```python
from build123d import *

# Parameters (mm, degrees)
SKETCH1_R           = 12.65
BOSS_EXTRUDE1_DEPTH = 4
SKETCH4_R           = 6
CUT_EXTRUDE3_DEPTH  = 0.5
SKETCH5_R           = 3
CUT_EXTRUDE4_DEPTH  = 1.5
FILLET1_R           = 0.5
FILLET2_R           = 0.5
FILLET3_R           = 0.5
SKETCH7_R           = 13.65
BOSS_EXTRUDE2_DEPTH = 1
SKETCH8_R           = 1.4
CUT_EXTRUDE6_DEPTH  = 20.941038087
CUT_EXTRUDE7_DEPTH  = 2.7
SKETCH16_R          = 1.65
CUT_EXTRUDE8_DEPTH  = 10


with BuildPart() as part:
    # Sketch1 → Boss-Extrude1 (new body)
    with BuildSketch(Plane(origin=(0, 0, 0), x_dir=(1, 0, 0), z_dir=(0, 1, 0))):
        with Locations(Location((0, 0, 0), (0, 0, 270))):
            Circle(SKETCH1_R)
    extrude(amount=BOSS_EXTRUDE1_DEPTH)

    # Sketch4 → Cut-Extrude3 (cut)
    with BuildSketch(Plane(origin=(0, 4, 0), x_dir=(1, 0, 0), z_dir=(0, 1, 0))):
        with Locations(Location((0, 0, 0), (0, 0, 270))):
            Circle(SKETCH4_R)
    extrude(amount=-CUT_EXTRUDE3_DEPTH, mode=Mode.SUBTRACT)

    # Sketch5 → Cut-Extrude4 (cut)
    with BuildSketch(Plane(origin=(0, 3.5, 0), x_dir=(1, 0, 0), z_dir=(0, 1, 0))):
        with Locations(Location((0, 0, 0), (0, 0, 270))):
            Circle(SKETCH5_R)
    extrude(amount=-CUT_EXTRUDE4_DEPTH, mode=Mode.SUBTRACT)

    # Fillet1
    fillet1_edges = [part.edges().sort_by_distance(p)[0] for p in [
        (0, 4, -6),
    ]]
    fillet(fillet1_edges, radius=FILLET1_R - 0.0001)  # a hair under: the kernel refuses the full size

    # Fillet2
    fillet2_edges = [part.edges().sort_by_distance(p)[0] for p in [
        (0, 3.5, -3),
    ]]
    fillet(fillet2_edges, radius=FILLET2_R)

    # Fillet3
    fillet3_edges = [part.edges().sort_by_distance(p)[0] for p in [
        (0, 4, -12.65),
    ]]
    fillet(fillet3_edges, radius=FILLET3_R)

    # Sketch7 → Boss-Extrude2 (add)
    with BuildSketch(Plane.XZ):
        with Locations(Location((0, 0, 0), (0, 0, 270))):
            Circle(SKETCH7_R)
    extrude(amount=BOSS_EXTRUDE2_DEPTH)

    # Sketch8 → Cut-Extrude6 (cut, through all)
    with BuildSketch(Plane(origin=(0, 4, 0), x_dir=(1, 0, 0), z_dir=(0, 1, 0))):
        with Locations(Location((0, 8, 0), (0, 0, 270))):
            Circle(SKETCH8_R)
        with Locations(Location((8, 0, 0), (0, 0, 270))):
            Circle(SKETCH8_R)
        with Locations(Location((0, -8, 0), (0, 0, 270))):
            Circle(SKETCH8_R)
        with Locations(Location((-8, 0, 0), (0, 0, 270))):
            Circle(SKETCH8_R)
    extrude(amount=-CUT_EXTRUDE6_DEPTH, mode=Mode.SUBTRACT)

    # Sketch15 → Cut-Extrude7 (cut)
    with BuildSketch(Plane(origin=(0, 4, 0), x_dir=(1, 0, 0), z_dir=(0, 1, 0))):
        Polygon((5.170983681, 0), (6.58549184, -2.45), (9.41450816, -2.45), (10.829016319, 0), (9.41450816, 2.45), (6.58549184, 2.45), align=None)
        Polygon((0, 5.170983681), (2.45, 6.58549184), (2.45, 9.41450816), (0, 10.829016319), (-2.45, 9.41450816), (-2.45, 6.58549184), align=None)
        Polygon((0, -5.170983681), (-2.45, -6.58549184), (-2.45, -9.41450816), (0, -10.829016319), (2.45, -9.41450816), (2.45, -6.58549184), align=None)
        Polygon((-5.170983681, 0), (-6.58549184, 2.45), (-9.41450816, 2.45), (-10.829016319, 0), (-9.41450816, -2.45), (-6.58549184, -2.45), align=None)
    extrude(amount=-CUT_EXTRUDE7_DEPTH, mode=Mode.SUBTRACT)

    # Sketch16 → Cut-Extrude8 (cut)
    with BuildSketch(Plane(origin=(0, 2, 0), x_dir=(1, 0, 0), z_dir=(0, 1, 0))):
        with Locations(Location((0, 0, 0), (0, 0, 270))):
            Circle(SKETCH16_R)
    extrude(amount=-CUT_EXTRUDE8_DEPTH, mode=Mode.SUBTRACT)


solid = part.part
```
Model file for the job. Use its own axes, mm. A direction names the side the tool comes from. Coordinates: 2 decimals unless noted, no trailing zeros. Loops run counter-clockwise (first coordinate to the right, second up) from the corner with the lowest first, then second, coordinate; pieces in that order, holes last. Notation, with made-up numbers: (-9, -35) - (39, -35) arc R20 cw to (39, -21) - close; hole circle Ø4 at (42.5, 30). An arc over 180 degrees is marked (long way). Answer as a JSON object with one key per item and string values. Group by question number.
(1) Flat gauge pins, fed straight in: pin 1 (1 mm diameter, centred on x = -3.5, y = 2.5, fed in from -Z); pin 2 (3 mm diameter, centred on x = -8, y = 3, fed in from +Z); pin 3 (1.4 mm diameter, centred on x = 7.5, y = 3, fed in from +Z); pin 4 (2 mm diameter, centred on x = 0, z = -8, fed in from -Y). Where does each tip first touch, or does it go through?
(2) Probe line 1 along X through (y, z) = (0.2, 0); line 2 along X through (y, z) = (-0.35, 0); line 3 along Z through (x, y) = (1.25, 1.1). List the from-to ranges inside material, lowest first.
(3) Cut at A-A (y = -0.4). Give the cut face in (x, z).
(4) Cut at B-B (x = -0.5). State how many separate pieces and enclosed holes the cut face has, then the cut area to 3 significant figures.
(5) Tool access for faces 1 (the face through (0.06, 0.17, 6.6)), 2 (the face through (10.13, 2.67, -1.21)): list every direction of +Z, -Z, +X, -X, +Y, -Y with a clear straight run to the whole face (end or side of a thin tool).
(6) Two-plate mould, pull along Z, no slides. Class faces 3 (the face through (-5, 4, 5)), 4 (the face through (-10.112, 2.669, -1.242)): released by +Z, released by -Z, zero draft, split by the parting line, or undercut.
Geometry says:
{
 "1": {"pin 1": "stops at z = -12.29", "pin 2": "stops at z = 10.85", "pin 3": "stops at z = 10.67", "pin 4": "passes through"},
 "2": {"line 1": "x = -12.65 to -9.4, -6.6 to -1.65, 1.65 to 6.6, 9.4 to 12.65", "line 2": "x = -13.65 to -9.4, -6.6 to -1.65, 1.65 to 6.6, 9.4 to 13.65", "line 3": "z = -12.59 to -8.63, -7.37 to -1.08, 1.08 to 7.37, 8.63 to 12.59"},
 "3": {"outline": "circle Ø27.3 at (0, 0); hole circle Ø2.8 at (-8, 0); hole circle Ø3.3 at (0, 0); hole circle Ø2.8 at (0, -8); hole circle Ø2.8 at (0, 8); hole circle Ø2.8 at (8, 0)"},
 "4": {"separate pieces": "4", "enclosed holes": "0", "area": "65.0 mm^2"},
 "5": {"face 1": "+Y, -Y", "face 2": "+Y"},
 "6": {"face 3": "zero draft", "face 4": "undercut"}
}
